Verification items for the finished model (mm, model axes). Face numbers are marked on the shaded views. A direction names the side the tool comes from. Give positions to 0.01 mm unless a question says otherwise; leave off trailing zeros. Loops run counter-clockwise (first coordinate to the right, second up) from the corner with the lowest first, then second, coordinate; pieces in that order, holes last. Notation, with made-up numbers: M 65.25,21 L 115.25,21 A22 ccw 115.25,57 Z; hole C 26,-23 d2. An arc over 180 degrees is marked long. Use a Markdown table: item, result.
from build123d import *

# Parameters (mm, degrees)
SKETCH1_R           = 2.5
BOSS_EXTRUDE1_DEPTH = 4
BOSS_EXTRUDE2_DEPTH = 4
BOSS_EXTRUDE3_DEPTH = 56
CUT_EXTRUDE1_REACH  = 154
FILLET1_R           = 2


with BuildPart() as part:
    # Sketch1 → Boss-Extrude1 (new body)
    with BuildSketch(Plane(origin=(0, 0, 0), x_dir=(1, 0, 0), z_dir=(0, 1, 0))):
        with BuildLine():
            Line((-51, -52), (-51, 52))
            ThreePointArc((-51, 52), (-43.970562748, 68.970562748), (-27, 76))
            Line((-27, 76), (27, 76))
            ThreePointArc((27, 76), (43.970562748, 68.970562748), (51, 52))
            Line((51, 52), (51, -52))
            ThreePointArc((51, -52), (43.970562748, -68.970562748), (27, -76))
            Line((27, -76), (-27, -76))
            ThreePointArc((-27, -76), (-43.970562748, -68.970562748), (-51, -52))
        make_face()
        with Locations((-36, 61)):
            Circle(SKETCH1_R, mode=Mode.SUBTRACT)
        with Locations((-36, -61)):
            Circle(SKETCH1_R, mode=Mode.SUBTRACT)
        with Locations((36, -61)):
            Circle(SKETCH1_R, mode=Mode.SUBTRACT)
        with Locations((36, 61)):
            Circle(SKETCH1_R, mode=Mode.SUBTRACT)
        with BuildLine():
            Line((-44, -36.928932188), (-44, 36.928932188))
            ThreePointArc((-44, 36.928932188), (-43.619397663, 38.84234935), (-42.535533906, 40.464466094))
            Line((-42.535533906, 40.464466094), (-15.464466094, 67.535533906))
            ThreePointArc((-15.464466094, 67.535533906), (-13.84234935, 68.619397663), (-11.928932188, 69))
            Line((-11.928932188, 69), (11.928932188, 69))
            ThreePointArc((11.928932188, 69), (13.84234935, 68.619397663), (15.464466094, 67.535533906))
            Line((15.464466094, 67.535533906), (42.535533906, 40.464466094))
            ThreePointArc((42.535533906, 40.464466094), (43.619397663, 38.84234935), (44, 36.928932188))
            Line((44, 36.928932188), (44, -36.928932188))
            ThreePointArc((44, -36.928932188), (43.619397663, -38.84234935), (42.535533906, -40.464466094))
            Line((42.535533906, -40.464466094), (15.464466094, -67.535533906))
            ThreePointArc((15.464466094, -67.535533906), (13.84234935, -68.619397663), (11.928932188, -69))
            Line((11.928932188, -69), (-11.928932188, -69))
            ThreePointArc((-11.928932188, -69), (-13.84234935, -68.619397663), (-15.464466094, -67.535533906))
            Line((-15.464466094, -67.535533906), (-42.535533906, -40.464466094))
            ThreePointArc((-42.535533906, -40.464466094), (-43.619397663, -38.84234935), (-44, -36.928932188))
        make_face(mode=Mode.SUBTRACT)
    extrude(amount=-BOSS_EXTRUDE1_DEPTH)

    # Sketch2 → Boss-Extrude2 (add)
    with BuildSketch(Plane(origin=(0, 0, 0), x_dir=(1, 0, 0), z_dir=(0, 1, 0))):
        with BuildLine():
            Line((-27, -76), (27, -76))
            ThreePointArc((27, -76), (43.970562748, -68.970562748), (51, -52))
            Line((51, -52), (51, 52))
            ThreePointArc((51, 52), (43.970562748, 68.970562748), (27, 76))
            Line((27, 76), (-27, 76))
            ThreePointArc((-27, 76), (-43.970562748, 68.970562748), (-51, 52))
            Line((-51, 52), (-51, -52))
            ThreePointArc((-51, -52), (-43.970562748, -68.970562748), (-27, -76))
        make_face()
        with BuildLine():
            Line((-50, 52), (-50, -52))
            ThreePointArc((-50, -52), (-43.263455967, -68.263455967), (-27, -75))
            Line((-27, -75), (27, -75))
            ThreePointArc((27, -75), (43.263455967, -68.263455967), (50, -52))
            Line((50, -52), (50, 52))
            ThreePointArc((50, 52), (43.263455967, 68.263455967), (27, 75))
            Line((27, 75), (-27, 75))
            ThreePointArc((-27, 75), (-43.263455967, 68.263455967), (-50, 52))
        make_face(mode=Mode.SUBTRACT)
    extrude(amount=BOSS_EXTRUDE2_DEPTH)

    # Sketch3 → Boss-Extrude3 (add)
    with BuildSketch(Plane.XZ.offset(4)):
        with BuildLine():
            Line((-51, -52), (-51, 52))
            ThreePointArc((-51, 52), (-43.970562748, 68.970562748), (-27, 76))
            Line((-27, 76), (27, 76))
            ThreePointArc((27, 76), (43.970562748, 68.970562748), (51, 52))
            Line((51, 52), (51, -52))
            ThreePointArc((51, -52), (43.970562748, -68.970562748), (27, -76))
            Line((27, -76), (-27, -76))
            ThreePointArc((-27, -76), (-43.970562748, -68.970562748), (-51, -52))
        make_face()
        with BuildLine():
            Line((-47, -52), (-47, 52))
            ThreePointArc((-47, 52), (-41.142135624, 66.142135624), (-27, 72))
            Line((-27, 72), (27, 72))
            ThreePointArc((27, 72), (41.142135624, 66.142135624), (47, 52))
            Line((47, 52), (47, -52))
            ThreePointArc((47, -52), (41.142135624, -66.142135624), (27, -72))
            Line((27, -72), (-27, -72))
            ThreePointArc((-27, -72), (-41.142135624, -66.142135624), (-47, -52))
        make_face(mode=Mode.SUBTRACT)
    extrude(amount=BOSS_EXTRUDE3_DEPTH)

    # Sketch4 → Cut-Extrude1 (cut, up to next)
    with BuildSketch(Plane.XY.offset(76), mode=Mode.PRIVATE) as cut_extrude1_sk1:
        with BuildLine():
            Line((5, -60), (-5, -60))
            Line((-5, -60), (-5, -50))
            ThreePointArc((-5, -50), (0, -45), (5, -50))
            Line((5, -50), (5, -60))
        make_face()
    cut_extrude1_tool1 = extrude(cut_extrude1_sk1.sketch, amount=-CUT_EXTRUDE1_REACH, mode=Mode.PRIVATE) & part.part
    add(cut_extrude1_tool1.solids().sort_by_distance((0, -52.991792, 76))[0], mode=Mode.SUBTRACT)

    # Fillet1
    fillet1_edges = [part.edges().sort_by_distance(p)[0] for p in [
        (-41.142135624, -4, -66.142135624),
        (0, -4, -72),
        (41.142135624, -4, -66.142135624),
        (47, -4, 0),
        (41.142135624, -4, 66.142135624),
        (0, -4, 72),
        (-41.142135624, -4, 66.142135624),
        (-47, -4, 0),
    ]]
    fillet(fillet1_edges, radius=FILLET1_R)


solid = part.part
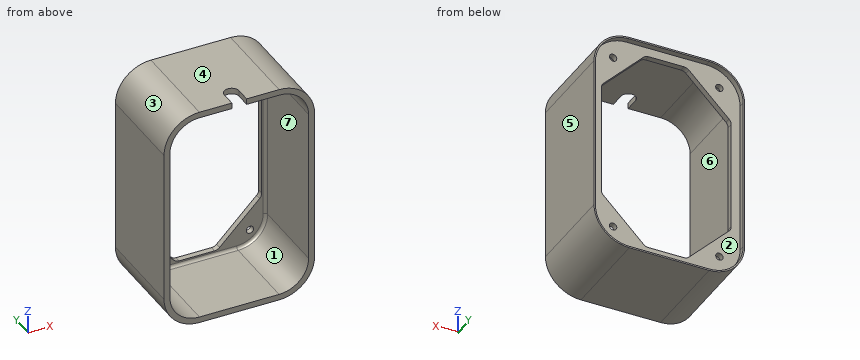
(1) Cross-section at A-A on x = 25. Record the cut outline in (y, z), then the cut area to 3 significant figures.
Results below:
| item | result |
|---|---|
| outline | M -60,-76 L 4,-76 L 4,-75 L 0,-75 L 0,-58 L -4,-58 L -4,-70 A2 cw -6,-72 L -60,-72 Z; M -60,72 L -6,72 A2 cw -4,70 L -4,58 L 0,58 L 0,75 L 4,75 L 4,76 L -60,76 Z |
| area | 602 mm^2 |
(2) Gauge pin test, flat ends, axial feed: P1, Ø1.2, axis at y = -53.5, z = 74.5, coming from the -X side; P2, Ø6, axis at x = -36, z = -61, coming from the -Y side; P3, Ø12, axis at y = -50.5, z = -59, coming from the +X side. Record the tip position at first contact, or that the pin passes through.
Results below:
| item | result |
|---|---|
| P1 | x = -36.82 |
| P2 | y = -4 |
| P3 | x = 50.98 |
(3) Cross-section at B-B on y = -25.5. Record the cut outline in (x, z), then the cut area to 3 significant figures.
Results below:
| item | result |
|---|---|
| outline | M -51,-52 A24 ccw -27,-76 L 27,-76 A24 ccw 51,-52 L 51,52 A24 ccw 27,76 L -27,76 A24 ccw -51,52 Z; hole M -47,-52 A20 ccw -27,-72 L 27,-72 A20 ccw 47,-52 L 47,52 A20 ccw 27,72 L -27,72 A20 ccw -47,52 Z |
| area | 1,820 mm^2 |
(4) Material ranges on line 1 (X direction, y = -45, z = -48); line 2 (X direction, y = -2.95, z = -61); line 3 (Z direction, x = 36, y = -1.65), recorded low to high.
Results below:
| item | result |
|---|---|
| line 1 | -51 to -47, 47 to 51 |
| line 2 | -49.25 to -38.5, -33.5 to -22, 22 to 33.5, 38.5 to 49.25 |
| line 3 | -74.25 to -63.5, -58.5 to -47, 47 to 58.5, 63.5 to 74.25 |
(5) Cross-section at C-C on z = -24. Record the cut outline in (x, y).
Results below:
| item | result |
|---|---|
| outline | M -51,-60 L -47,-60 L -47,-6 A2 cw -45,-4 L -44,-4 L -44,0 L -50,0 L -50,4 L -51,4 Z; M 44,-4 L 45,-4 A2 cw 47,-6 L 47,-60 L 51,-60 L 51,4 L 50,4 L 50,0 L 44,0 Z |
(6) Draft check along X on the marked faces 4, 5, 6 and 7. Enter one of: +X half, -X half, draft (parallel to the pull), parting line (faces both ways), or undercut.
Results below:
| item | result |
|---|---|
| face 4 | draft |
| face 5 | +X half |
| face 6 | undercut |
| face 7 | undercut |
(7) Set-up check for the marked faces 1, 2 and 3: record each of +Z, -Z, +X, -X, +Y, -Y from which the full face is reachable in a straight line by a thin tool's end or side.
Results below:
| item | result |
|---|---|
| face 1 | -Y |
| face 2 | +Y |
| face 3 | +Z, -X, +Y, -Y |
(8) Cross-section at D-D on y = -54. Record the cut outline in (x, z).
Results below:
| item | result |
|---|---|
| outline | M -51,-52 A24 ccw -27,-76 L 27,-76 A24 ccw 51,-52 L 51,52 A24 ccw 27,76 L 5,76 L 5,72 L 27,72 A20 cw 47,52 L 47,-52 A20 cw 27,-72 L -27,-72 A20 cw -47,-52 L -47,52 A20 cw -27,72 L -5,72 L -5,76 L -27,76 A24 ccw -51,52 Z |
